Design review of the part built by this model. Coordinates are the model's own, in mm. A direction names the side the tool comes from. Give positions to 0.01 mm unless a question says otherwise; leave off trailing zeros. Write each loop counter-clockwise with the first axis right and the second up, starting at its lowest first coordinate (ties: lowest second). Pieces come first, ordered by that corner, then holes. Notation, with made-up numbers: M -2.75,-21 L 24.25,-21 A17 cw 24.25,-12 Z; hole C 62,-23 d9. An arc over 180 degrees is marked long. Answer in a Markdown table with one row per item.
```python
from build123d import *

# Parameters (mm, degrees)
SKETCH_1_W          = 47.8
SKETCH_1_H          = 7.8
EXTRUDE_1_DEPTH     = 3.2
SKETCH_2_R          = 2.4
EXTRUDE_2_DEPTH     = 1.7
SKETCH_3_R          = 2.5
CUT_EXTRUDE_1_DEPTH = 1.8


with BuildPart() as part:
    # Эскиз1 → Бобышка-Вытянуть1 (new body)
    with BuildSketch(Plane(origin=(0, 0, 0), x_dir=(1, 0, 0), z_dir=(0, 1, 0))):
        Rectangle(SKETCH_1_W, SKETCH_1_H)
    extrude(amount=EXTRUDE_1_DEPTH)

    # Эскиз2 → Бобышка-Вытянуть2 (add)
    with BuildSketch(Plane(origin=(0, 3.2, 0), x_dir=(1, 0, 0), z_dir=(0, 1, 0))):
        with Locations(Location((-20, 0, 0), (0, 0, 270))):
            Circle(SKETCH_2_R)
        with Locations(Location((-12, 0, 0), (0, 0, 270))):
            Circle(SKETCH_2_R)
        with Locations(Location((-4, 0, 0), (0, 0, 270))):
            Circle(SKETCH_2_R)
        with Locations(Location((4, 0, 0), (0, 0, 270))):
            Circle(SKETCH_2_R)
        with Locations(Location((12, 0, 0), (0, 0, 270))):
            Circle(SKETCH_2_R)
        with Locations(Location((20, 0, 0), (0, 0, 270))):
            Circle(SKETCH_2_R)
    extrude(amount=EXTRUDE_2_DEPTH)

    # Эскиз3 → Вырез-Вытянуть1 (cut)
    with BuildSketch(Plane.XZ):
        with Locations(Location((-20, 0, 0), (0, 0, 270))):
            Circle(SKETCH_3_R)
        with Locations(Location((-12, 0, 0), (0, 0, 270))):
            Circle(SKETCH_3_R)
        with Locations(Location((-4, 0, 0), (0, 0, 270))):
            Circle(SKETCH_3_R)
        with Locations(Location((4, 0, 0), (0, 0, 270))):
            Circle(SKETCH_3_R)
        with Locations(Location((12, 0, 0), (0, 0, 270))):
            Circle(SKETCH_3_R)
        with Locations(Location((20, 0, 0), (0, 0, 270))):
            Circle(SKETCH_3_R)
    extrude(amount=-CUT_EXTRUDE_1_DEPTH, mode=Mode.SUBTRACT)


solid = part.part
```
1) Add section A-A (x = -4). Write out the cut boundary in (y, z).
Geometry says:
| item | result |
|---|---|
| outline | M 0,-3.9 L 3.2,-3.9 L 3.2,-2.4 L 4.9,-2.4 L 4.9,2.4 L 3.2,2.4 L 3.2,3.9 L 0,3.9 L 0,2.5 L 1.8,2.5 L 1.8,-2.5 L 0,-2.5 Z |
2) The part is to be moulded in two halves that separate along Z. For faces 1 (the face through (6.48, 0.89, 0.33)), 2 (the face through (12, 1.8, 0)), 3 (the face through (0, 2, 3.9)), 4 (the face through (20, 4.9, 0)), say which applies: released by +Z, released by -Z, zero draft, split by the parting line, or undercut.
Geometry says:
| item | result |
|---|---|
| face 1 | undercut |
| face 2 | undercut |
| face 3 | released by +Z |
| face 4 | zero draft |
3) Insertion check: P1, Ø1.5, axis at x = -12, z = 0, coming from the -Y side; P2, Ø2, axis at x = 1, z = 2.5, coming from the +Y side. Each pin has a flat end and moves straight along its axis. Give the tip position at first contact, or say it passes through.
Geometry says:
| item | result |
|---|---|
| P1 | y = 1.8 |
| P2 | y = 3.2 |
4) For faces 5 (the face through (-20, 4.9, 0)), 6 (the face through (-22.343, 4.038, -0.52)), 7 (the face through (4, 1.8, 0)), list the 3-axis set-ups (+Z, -Z, +X, -X, +Y, -Y) from which the entire face can be reached by the end or side of a thin tool; tool diameter is ignored.
Geometry says:
| item | result |
|---|---|
| face 5 | +Z, -Z, +X, -X, +Y |
| face 6 | +Y |
| face 7 | -Y |
5) Add section D-D (x = 7.5). Write out the cut boundary in (y, z).
Geometry says:
| item | result |
|---|---|
| outline | M 0,-3.9 L 3.2,-3.9 L 3.2,3.9 L 0,3.9 Z |
6) Add section B-B (y = 4.15). Write out the cut boundary in (x, z).
Geometry says:
| item | result |
|---|---|
| outline | C -20,0 d4.8; C -12,0 d4.8; C -4,0 d4.8; C 4,0 d4.8; C 12,0 d4.8; C 20,0 d4.8 |
7) Add section C-C (x = -13.5). Write out the cut boundary in (y, z), and give its area (3 significant figures).
Geometry says:
| item | result |
|---|---|
| outline | M 0,-3.9 L 3.2,-3.9 L 3.2,-1.87 L 4.9,-1.87 L 4.9,1.87 L 3.2,1.87 L 3.2,3.9 L 0,3.9 L 0,2 L 1.8,2 L 1.8,-2 L 0,-2 Z |
| area | 24.1 mm^2 |
8) To check wall thickness, follow probe 1 along X at (y, z) = (4.2, -0.5); probe 2 along X at (y, z) = (3.5, -1); probe 3 along Y at (x, z) = (-8, 1.5). State the ranges of each line that lie inside material, in increasing order. Write a range as [from, to].
Geometry says:
| item | result |
|---|---|
| probe 1 | [-22.35, -17.65], [-14.35, -9.65], [-6.35, -1.65], [1.65, 6.35], [9.65, 14.35], [17.65, 22.35] |
| probe 2 | [-22.18, -17.82], [-14.18, -9.82], [-6.18, -1.82], [1.82, 6.18], [9.82, 14.18], [17.82, 22.18] |
| probe 3 | [0, 3.2] |
